For this review, use the dimensioned drawing (mm, ordinates from the lowest corner) and the shaded views. Coordinates: 2 decimals unless noted, no trailing zeros. Order: outer loops, then holes, each group sorted by start corner. A loop starts at its lowest first (then second) coordinate and runs counter-clockwise, first axis right, second up. Notation, with made-up numbers: (4, 74.25) -> (14, 74.25) arc R25 ccw to (14, 105.25) -> close; hole circle Ø6 at (35.5, 13.25). An arc over 180 degrees is marked (long way). Return JSON: item names as keys, results as strings. Group by question number.
Item 1: Take a section at C-C (z = 143). Write out the cut boundary in (x, y).
Item 2: Insertion check: pin 1 (3 mm diameter, centred on y = 3.5, z = 151.5, fed in from -X). The pin has a flat end and moves straight along its axis. Give the tip position at first contact, or say it passes through.
Item 3: Take a section at A-A (z = 173.5). Write out the cut boundary in (x, y), then the cut area to 3 significant figures.
Item 4: Take a section at B-B (y = 2). Write out the cut boundary in (x, z), then the cut area to 3 significant figures.
Item 5: For line 1 along X through (y, z) = (1.75, 146.5); line 2 along X through (y, z) = (1.5, 148.5); line 3 along Z through (x, y) = (676.5, 1), list the stretches that pass through material, from the lowest coordinate up.
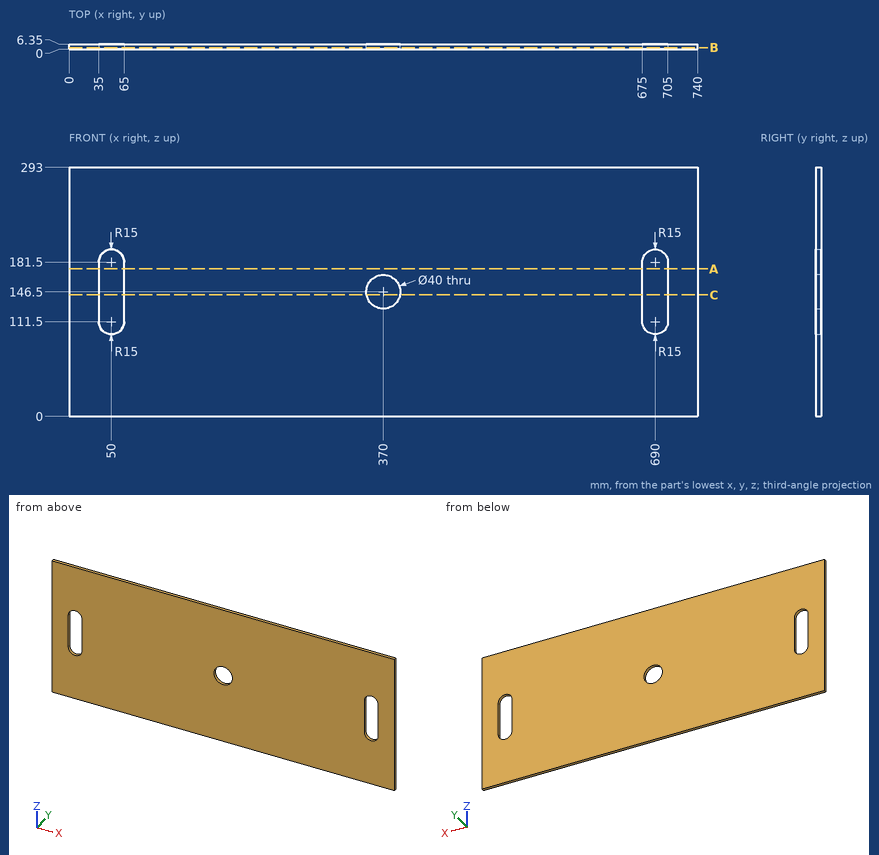
Findings below:
{
 "1": {"outline": "(0, 0) -> (35, 0) -> (35, 6.35) -> (0, 6.35) -> close; (65, 0) -> (350.31, 0) -> (350.31, 6.35) -> (65, 6.35) -> close; (389.69, 0) -> (675, 0) -> (675, 6.35) -> (389.69, 6.35) -> close; (705, 0) -> (740, 0) -> (740, 6.35) -> (705, 6.35) -> close"},
 "2": {"pin 1": "stops at x = 0"},
 "3": {"outline": "(0, 0) -> (35, 0) -> (35, 6.35) -> (0, 6.35) -> close; (65, 0) -> (675, 0) -> (675, 6.35) -> (65, 6.35) -> close; (705, 0) -> (740, 0) -> (740, 6.35) -> (705, 6.35) -> close", "area": "4,320 mm2"},
 "4": {"outline": "(0, 0) -> (740, 0) -> (740, 293) -> (0, 293) -> close; hole (35, 111.5) arc R15 ccw to (65, 111.5) -> (65, 181.5) arc R15 ccw to (35, 181.5) -> close; hole circle Ø40 at (370, 146.5); hole (675, 111.5) arc R15 ccw to (705, 111.5) -> (705, 181.5) arc R15 ccw to (675, 181.5) -> close", "area": "210,000 mm2"},
 "5": {"line 1": "x = 0 to 35, 65 to 350, 390 to 675, 705 to 740", "line 2": "x = 0 to 35, 65 to 350.1, 389.9 to 675, 705 to 740", "line 3": "z = 0 to 104.96, 188.04 to 293"}
}
